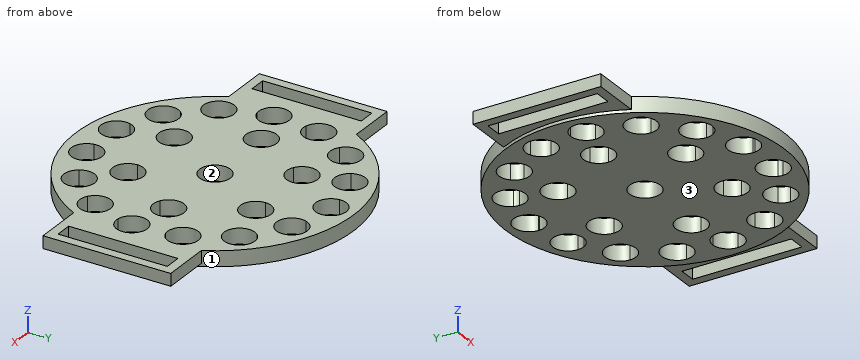
```python
from build123d import *

# Parameters (mm, degrees)
F0_R     = 45.2030485361
F0_R_2   = 5
F1_DEPTH = 5
F2_W     = 5.5
F2_H     = 35.5464573561
F3_DEPTH = 4


with BuildPart() as f1:
    # F0 (on Top) → F1 (new body)
    with BuildSketch(Plane.XY):
        Circle(F0_R)
        with BuildLine():
            ThreePointArc((36.8300827761, 7.0565574258), (37.2595815037, 4.2395266444), (37.4739316415, 1.3980154974))
            ThreePointArc((37.4739316415, 1.3980154974), (40.9139869844, -0.1166869301), (42.3268174051, -3.5998197741))
            ThreePointArc((42.3268174051, -3.5998197741), (40.5630566958, -7.4112178448), (36.5161153038, -8.5336582497))
            ThreePointArc((36.5161153038, -8.5336582497), (35.762692272, -11.2818367947), (34.8027641615, -13.9648704513))
            ThreePointArc((34.8027641615, -13.9648704513), (36.8685312345, -15.8095798691), (37.6355658781, -18.470783411))
            ThreePointArc((37.6355658781, -18.470783411), (35.0086513584, -22.8717452721), (29.8881797569, -22.6483268879))
            ThreePointArc((29.8881797569, -22.6483268879), (28.0821086525, -24.8524681597), (26.1138825848, -26.9131034321))
            ThreePointArc((26.1138825848, -26.9131034321), (26.9950887613, -28.4250139192), (27.3013285259, -30.1479807944))
            ThreePointArc((27.3013285259, -30.1479807944), (23.7075449731, -34.9461632944), (18.0923064045, -32.8468940536))
            ThreePointArc((18.0923064045, -32.8468940536), (15.5458733291, -34.1258820023), (12.909673472, -35.2078163317))
            ThreePointArc((12.909673472, -35.2078163317), (13.0604041393, -35.9028901243), (13.1109888705, -36.6123184126))
            ThreePointArc((13.1109888705, -36.6123184126), (8.4888778779, -41.5980179521), (3.1681089112, -37.3659348328))
            ThreePointArc((3.1681089112, -37.3659348328), (0.3216152773, -37.4986208228), (-2.5267354648, -37.4147779345))
            ThreePointArc((-2.5267354648, -37.4147779345), (-8.4793897063, -41.6455273734), (-12.3038833941, -35.4240660205))
            ThreePointArc((-12.3038833941, -35.4240660205), (-14.9582529778, -34.3875074388), (-17.5262488851, -33.1523845299))
            ThreePointArc((-17.5262488851, -33.1523845299), (-24.6850699528, -34.5962038586), (-25.6484224833, -27.3570543758))
            ThreePointArc((-25.6484224833, -27.3570543758), (-27.6517034015, -25.3304816179), (-29.4953146521, -23.1576426601))
            ThreePointArc((-29.4953146521, -23.1576426601), (-36.6224773476, -21.5648824), (-34.5581163166, -14.5597594984))
            ThreePointArc((-34.5581163166, -14.5597594984), (-35.5639230993, -11.8935854051), (-36.3643725593, -9.1587339938))
            ThreePointArc((-36.3643725593, -9.1587339938), (-42.2275257042, -4.8047968637), (-37.492397888, 0.7550500675))
            ThreePointArc((-37.492397888, 0.7550500675), (-37.3268174051, 3.5998197741), (-36.945700091, 6.4238029846))
            ThreePointArc((-36.945700091, 6.4238029846), (-40.5310512416, 12.7860817006), (-33.943903257, 15.9393046173))
            ThreePointArc((-33.943903257, 15.9393046173), (-32.6355658781, 18.470783411), (-31.1387804359, 20.8956060684))
            ThreePointArc((-31.1387804359, 20.8956060684), (-31.8263898062, 28.166130581), (-24.526199382, 28.3675085947))
            ThreePointArc((-24.526199382, 28.3675085947), (-22.3013285259, 30.1479807944), (-19.9476827564, 31.7543690325))
            ThreePointArc((-19.9476827564, 31.7543690325), (-17.6186564397, 38.6759996026), (-10.8676928205, 35.8907126254))
            ThreePointArc((-10.8676928205, 35.8907126254), (-8.1109888705, 36.6123184126), (-5.3074495093, 37.1225131114))
            ThreePointArc((-5.3074495093, 37.1225131114), (-0.5098024711, 42.4950781258), (4.6783847227, 37.4986208228))
            ThreePointArc((4.6783847227, 37.4986208228), (4.6762722357, 37.3532922036), (4.6699365597, 37.2080863863))
            ThreePointArc((4.6699365597, 37.2080863863), (7.4818144468, 36.7460535648), (10.2504899745, 36.0718374259))
            ThreePointArc((10.2504899745, 36.0718374259), (15.8130000116, 39.3139064795), (19.9582529778, 34.3875074388))
            ThreePointArc((19.9582529778, 34.3875074388), (19.8167091384, 33.2062353552), (19.4000914836, 32.0918439861))
            ThreePointArc((19.4000914836, 32.0918439861), (21.780944076, 30.5260622282), (24.036026619, 28.7840133471))
            ThreePointArc((24.036026619, 28.7840133471), (29.5120281161, 29.9715151188), (32.6517034015, 25.3304816179))
            ThreePointArc((32.6517034015, 25.3304816179), (32.1583903621, 23.1648933284), (30.7757943457, 21.4266302155))
            ThreePointArc((30.7757943457, 21.4266302155), (32.3139506008, 19.0278374118), (33.6655159007, 16.5191718661))
            ThreePointArc((33.6655159007, 16.5191718661), (38.3485203778, 16.046417932), (40.5639230993, 11.8935854051))
            ThreePointArc((40.5639230993, 11.8935854051), (39.5218770141, 8.8383275096), (36.8300827761, 7.0565574258))
        make_face(mode=Mode.SUBTRACT)
        with BuildLine():
            ThreePointArc((36.5161153038, -8.5336582497), (32.3499084178, -3.1198438042), (37.4739316415, 1.3980154974))
            ThreePointArc((37.4739316415, 1.3980154974), (37.2595815037, 4.2395266444), (36.8300827761, 7.0565574258))
            ThreePointArc((36.8300827761, 7.0565574258), (30.822066686, 10.3077740177), (33.6655159007, 16.5191718661))
            ThreePointArc((33.6655159007, 16.5191718661), (32.3139506008, 19.0278374118), (30.7757943457, 21.4266302155))
            ThreePointArc((30.7757943457, 21.4266302155), (23.9648096146, 21.9530840689), (24.036026619, 28.7840133471))
            ThreePointArc((24.036026619, 28.7840133471), (21.780944076, 30.5260622282), (19.4000914836, 32.0918439861))
            ThreePointArc((19.4000914836, 32.0918439861), (12.9638192474, 29.802506447), (10.2504899745, 36.0718374259))
            ThreePointArc((10.2504899745, 36.0718374259), (7.4818144468, 36.7460535648), (4.6699365597, 37.2080863863))
            ThreePointArc((4.6699365597, 37.2080863863), (-0.2787332403, 32.4988047131), (-5.3074495093, 37.1225131114))
            ThreePointArc((-5.3074495093, 37.1225131114), (-8.1109888705, 36.6123184126), (-10.8676928205, 35.8907126254))
            ThreePointArc((-10.8676928205, 35.8907126254), (-10.6269861306, 35.0228484054), (-10.5458733291, 34.1258820023))
            ThreePointArc((-10.5458733291, 34.1258820023), (-14.3229765911, 29.2777355969), (-19.9476827564, 31.7543690325))
            ThreePointArc((-19.9476827564, 31.7543690325), (-22.3013285259, 30.1479807944), (-24.526199382, 28.3675085947))
            ThreePointArc((-24.526199382, 28.3675085947), (-23.4572007425, 26.7525278492), (-23.0821086525, 24.8524681597))
            ThreePointArc((-23.0821086525, 24.8524681597), (-25.8779488258, 20.3645199137), (-31.1387804359, 20.8956060684))
            ThreePointArc((-31.1387804359, 20.8956060684), (-32.6355658781, 18.470783411), (-33.943903257, 15.9393046173))
            ThreePointArc((-33.943903257, 15.9393046173), (-31.6338943189, 14.1019480447), (-30.762692272, 11.2818367947))
            ThreePointArc((-30.762692272, 11.2818367947), (-32.6736017177, 7.3502315821), (-36.945700091, 6.4238029846))
            ThreePointArc((-36.945700091, 6.4238029846), (-37.3268174051, 3.5998197741), (-37.492397888, 0.7550500675))
            ThreePointArc((-37.492397888, 0.7550500675), (-33.8073417903, -0.6226162279), (-32.2595815037, -4.2395266444))
            ThreePointArc((-32.2595815037, -4.2395266444), (-33.4205683022, -7.4429588099), (-36.3643725593, -9.1587339938))
            ThreePointArc((-36.3643725593, -9.1587339938), (-35.5639230993, -11.8935854051), (-34.5581163166, -14.5597594984))
            ThreePointArc((-34.5581163166, -14.5597594984), (-29.6891485681, -14.7722041699), (-27.3139506008, -19.0278374118))
            ThreePointArc((-27.3139506008, -19.0278374118), (-27.8927980506, -21.3630911728), (-29.4953146521, -23.1576426601))
            ThreePointArc((-29.4953146521, -23.1576426601), (-27.6517034015, -25.3304816179), (-25.6484224833, -27.3570543758))
            ThreePointArc((-25.6484224833, -27.3570543758), (-20.0982961682, -25.8176977544), (-16.780944076, -30.5260622282))
            ThreePointArc((-16.780944076, -30.5260622282), (-16.9708777586, -31.8910757896), (-17.5262488851, -33.1523845299))
            ThreePointArc((-17.5262488851, -33.1523845299), (-14.9582529778, -34.3875074388), (-12.3038833941, -35.4240660205))
            ThreePointArc((-12.3038833941, -35.4240660205), (-6.8148604516, -31.7907359798), (-2.4818144468, -36.7460535648))
            ThreePointArc((-2.4818144468, -36.7460535648), (-2.4930573415, -37.0811692838), (-2.5267354648, -37.4147779345))
            ThreePointArc((-2.5267354648, -37.4147779345), (0.3216152773, -37.4986208228), (3.1681089112, -37.3659348328))
            ThreePointArc((3.1681089112, -37.3659348328), (7.0295236877, -31.7306759576), (12.909673472, -35.2078163317))
            ThreePointArc((12.909673472, -35.2078163317), (15.5458733291, -34.1258820023), (18.0923064045, -32.8468940536))
            ThreePointArc((18.0923064045, -32.8468940536), (19.3278180558, -26.1282500218), (26.1138825848, -26.9131034321))
            ThreePointArc((26.1138825848, -26.9131034321), (28.0821086525, -24.8524681597), (29.8881797569, -22.6483268879))
            ThreePointArc((29.8881797569, -22.6483268879), (28.2841570943, -16.0080122895), (34.8027641615, -13.9648704513))
            ThreePointArc((34.8027641615, -13.9648704513), (35.762692272, -11.2818367947), (36.5161153038, -8.5336582497))
        make_face()
        with BuildLine():
            ThreePointArc((-14.4934291692, 16.4431016591), (-14.4934291692, 25.103355697), (-6.9934291692, 20.7732286781))
            Line((-6.9934291692, 20.7732286781), (6.9934291692, 20.7732286781))
            ThreePointArc((6.9934291692, 20.7732286781), (11.9934291692, 25.7732286781), (16.9934291692, 20.7732286781))
            ThreePointArc((16.9934291692, 20.7732286781), (16.3235561881, 18.2732286781), (14.4934291692, 16.4431016591))
            Line((14.4934291692, 16.4431016591), (21.4868583384, 4.3301270189))
            ThreePointArc((21.4868583384, 4.3301270189), (26.4868583384, 4.3301270189), (28.9868583384, 0))
            ThreePointArc((28.9868583384, 0), (26.4868583384, -4.3301270189), (21.4868583384, -4.3301270189))
            Line((21.4868583384, -4.3301270189), (14.4934291692, -16.4431016591))
            ThreePointArc((14.4934291692, -16.4431016591), (16.3235561881, -18.2732286781), (16.9934291692, -20.7732286781))
            ThreePointArc((16.9934291692, -20.7732286781), (11.9934291692, -25.7732286781), (6.9934291692, -20.7732286781))
            Line((6.9934291692, -20.7732286781), (-6.9934291692, -20.7732286781))
            ThreePointArc((-6.9934291692, -20.7732286781), (-14.4934291692, -25.103355697), (-14.4934291692, -16.4431016591))
            Line((-14.4934291692, -16.4431016591), (-21.4868583384, -4.3301270189))
            ThreePointArc((-21.4868583384, -4.3301270189), (-28.9868583384, 0), (-21.4868583384, 4.3301270189))
            Line((-21.4868583384, 4.3301270189), (-14.4934291692, 16.4431016591))
        make_face(mode=Mode.SUBTRACT)
        with BuildLine():
            Line((6.9934291692, 20.7732286781), (-6.9934291692, 20.7732286781))
            ThreePointArc((-6.9934291692, 20.7732286781), (-9.4934291692, 16.4431016591), (-14.4934291692, 16.4431016591))
            Line((-14.4934291692, 16.4431016591), (-21.4868583384, 4.3301270189))
            ThreePointArc((-21.4868583384, 4.3301270189), (-19.6567313195, 2.5), (-18.9868583384, 0))
            ThreePointArc((-18.9868583384, 0), (-19.6567313195, -2.5), (-21.4868583384, -4.3301270189))
            Line((-21.4868583384, -4.3301270189), (-14.4934291692, -16.4431016591))
            ThreePointArc((-14.4934291692, -16.4431016591), (-9.4934291692, -16.4431016591), (-6.9934291692, -20.7732286781))
            Line((-6.9934291692, -20.7732286781), (6.9934291692, -20.7732286781))
            ThreePointArc((6.9934291692, -20.7732286781), (9.4934291692, -16.4431016591), (14.4934291692, -16.4431016591))
            Line((14.4934291692, -16.4431016591), (21.4868583384, -4.3301270189))
            ThreePointArc((21.4868583384, -4.3301270189), (18.9868583384, 0), (21.4868583384, 4.3301270189))
            Line((21.4868583384, 4.3301270189), (14.4934291692, 16.4431016591))
            ThreePointArc((14.4934291692, 16.4431016591), (9.4934291692, 16.4431016591), (6.9934291692, 20.7732286781))
        make_face()
        Circle(F0_R_2, mode=Mode.SUBTRACT)
    extrude(amount=F1_DEPTH)

    # F2 (on face) → F3 (join)
    with BuildSketch(Plane.XY.offset(5)):
        with BuildLine():
            ThreePointArc((-40.1470866595, -20.7732286781), (-45.2030485361, 0), (-40.1470866595, 20.7732286781))
            Line((-40.1470866595, 20.7732286781), (-55.9934291692, 20.7732286781))
            Line((-55.9934291692, 20.7732286781), (-55.9934291692, -20.7732286781))
            Line((-55.9934291692, -20.7732286781), (-40.1470866595, -20.7732286781))
        make_face()
        with Locations((-50.2434291692, 0)):
            Rectangle(F2_W, F2_H, mode=Mode.SUBTRACT)
        with BuildLine():
            ThreePointArc((40.1470866595, 20.7732286781), (43.9208737607, 10.6898290469), (45.2030485361, 0))
            ThreePointArc((45.2030485361, 0), (43.9208737607, -10.6898290469), (40.1470866595, -20.7732286781))
            Line((40.1470866595, -20.7732286781), (55.9934291692, -20.7732286781))
            Line((55.9934291692, -20.7732286781), (55.9934291692, 20.7732286781))
            Line((55.9934291692, 20.7732286781), (40.1470866595, 20.7732286781))
        make_face()
        with Locations((50.2434291692, 0)):
            Rectangle(F2_W, F2_H, mode=Mode.SUBTRACT)
    extrude(amount=-F3_DEPTH)


solid = f1.part
```
Here's how the part is built. I have some questions about the finished solid (model axes, mm). Face numbers are marked on the shaded views. Give positions to 0.01 mm unless a question says otherwise; leave off trailing zeros. Order: outer loops, then holes, each group sorted by start corner. A loop starts at its lowest first (then second) coordinate and runs counter-clockwise, first axis right, second up. Notation, with made-up numbers: (-12.75, 60.25) -> (14.25, 60.25) arc R11 cw to (14.25, 72.25) -> close; hole circle Ø6 at (-19, 32). An arc over 180 degrees is marked (long way). Use CSV: the item, a comma, the result in double quotes. Start each with the question number.
Item 1: Suppose I cut it at A-A (x = 0). List the corners of the cut face in (y, z) for me, and give its area (3 significant figures).
Item 2: I'm going to push flat-ended pins straight in: P1, Ø9, axis at x = 0, y = 0, coming from the -Z side; P2, Ø1, axis at x = 5.5, z = 4, coming from the -Y side; P3, Ø2, axis at x = 14, z = 1.5, coming from the +Y side; P4, Ø2, axis at x = -46, z = 3.5, coming from the -Y side. Where does each tip first touch, or does it pass through?
Item 3: Suppose I cut it at C-C (z = 3.8). Give the number of separate pieces and of enclosed holes in the cut face, and give its area (3 significant figures).
Item 4: Suppose I cut it at B-B (y = -11). List the corners of the cut face in (x, z) for me.
Item 5: Thinking about a two-plate mould opening in Y: for the marked faces 1, 2 and 3, which applies, pulls with the +Y half, pulls with the -Y half, needs draft (parallel to the pull), parting line crosses it, or undercut?
Item 6: If I drill on probe 1 along Y at (x, z) = (0, 2.9); probe 2 along X at (y, z) = (-33, 1.75); probe 3 along X at (y, z) = (14, 1.5), over which ranges is the centre line in solid material (lowest first)? Write a range as [from, to].
Answer block:
1,outline,"(-45.2, 0) -> (-5, 0) -> (-5, 5) -> (-45.2, 5) -> close; (5, 0) -> (32.51, 0) -> (32.51, 5) -> (5, 5) -> close; (42.49, 0) -> (45.2, 0) -> (45.2, 5) -> (42.49, 5) -> close"
1,area,"352 mm^2"
2,P1,"passes through"
2,P2,"stops at y = -44.93"
2,P3,"stops at y = 43.29"
2,P4,"stops at y = -20.77"
3,separate pieces,"1"
3,enclosed holes,"24"
3,area,"5,330 mm^2"
4,outline,"(-55.99, 1) -> (-52.99, 1) -> (-52.99, 5) -> (-55.99, 5) -> close; (-47.49, 1) -> (-43.84, 1) -> (-43.84, 0) -> (43.84, 0) -> (43.84, 1) -> (47.49, 1) -> (47.49, 5) -> (-47.49, 5) -> close; (52.99, 1) -> (55.99, 1) -> (55.99, 5) -> (52.99, 5) -> close"
5,face 1,"parting line crosses it"
5,face 2,"undercut"
5,face 3,"needs draft"
6,probe 1,"y = [-45.2, -5], [5, 32.51], [42.49, 45.2]"
6,probe 2,"x = [-30.89, -26.13], [-17.44, -10.79], [-4.17, 4.65], [11.57, 18.19], [26.41, 30.89]"
6,probe 3,"x = [-55.99, -52.99], [-47.49, -39.96], [-31.57, 31.03], [40.1, 47.49], [52.99, 55.99]"
